from build123d import *

# Parameters (mm, degrees)
CROQUIS1_W              = 5
CROQUIS1_H              = 35
SALIENTE_EXTRUIR2_DEPTH = 5


with BuildPart() as part:
    # Croquis1 → Saliente-Extruir2 (new body)
    with BuildSketch(Plane(origin=(0, 0, 0), x_dir=(1, 0, 0), z_dir=(0, 1, 0))):
        with BuildLine():
            Line((-40, -25), (40, -25))
            ThreePointArc((40, -25), (47.071067812, -22.071067812), (50, -15))
            Line((50, -15), (50, 15))
            ThreePointArc((50, 15), (47.071067812, 22.071067812), (40, 25))
            Line((40, 25), (-40, 25))
            ThreePointArc((-40, 25), (-47.071067812, 22.071067812), (-50, 15))
            Line((-50, 15), (-50, -15))
            ThreePointArc((-50, -15), (-47.071067812, -22.071067812), (-40, -25))
        make_face()
        with Locations((-45, 0)):
            Rectangle(CROQUIS1_W, CROQUIS1_H, mode=Mode.SUBTRACT)
        with Locations((45, 0)):
            Rectangle(CROQUIS1_W, CROQUIS1_H, mode=Mode.SUBTRACT)
    extrude(amount=SALIENTE_EXTRUIR2_DEPTH)


solid = part.part
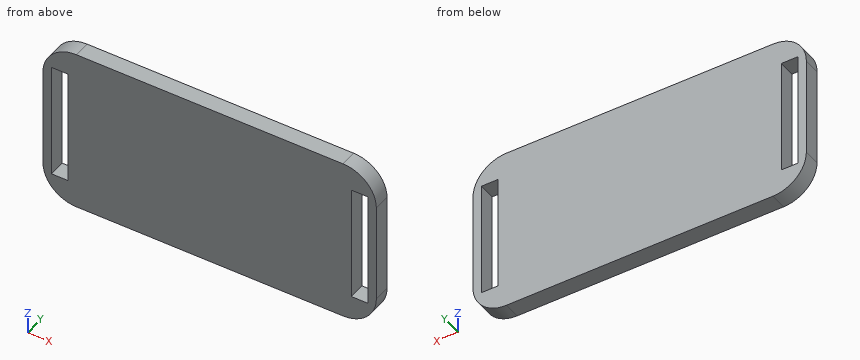
Input: part model. Units: mm. Frame: model coordinates. Coordinates: 2 decimals unless noted, no trailing zeros. Order: outer loops, then holes, each group sorted by start corner. A loop starts at its lowest first (then second) coordinate and runs counter-clockwise, first axis right, second up. Notation, with made-up numbers: M 13.25,46 L 57.25,46 A9 cw 57.25,61 Z; hole C -5,70.25 d10. An arc over 180 degrees is marked long. Answer in a Markdown table with one row per item.
(1) Material intervals for line 1 (X direction, y = 2.6, z = 2); line 2 (X direction, y = 1.9, z = 17); line 3 (Z direction, x = 43.5, y = 4.85), sorted ascending. Write a range as [from, to].
Numbers:
| item | result |
|---|---|
| line 1 | x = [-50, -47.5], [-42.5, 42.5], [47.5, 50] |
| line 2 | x = [-49.8, -47.5], [-42.5, 42.5], [47.5, 49.8] |
| line 3 | z = [-24.37, -17.5], [17.5, 24.37] |
(2) Section query C-C, the plane z = -16.5. Output: boundary loops of the cut face in (x, y), plus the area to 3 significant figures.
Numbers:
| item | result |
|---|---|
| outline | M -49.89,0 L -47.5,0 L -47.5,5 L -49.89,5 Z; M -42.5,0 L 42.5,0 L 42.5,5 L -42.5,5 Z; M 47.5,0 L 49.89,0 L 49.89,5 L 47.5,5 Z |
| area | 449 mm^2 |
(3) Section query B-B, the plane y = 2.2. Output: boundary loops of the cut face in (x, z), plus the area to 3 significant figures.
Numbers:
| item | result |
|---|---|
| outline | M -50,-15 A10 ccw -40,-25 L 40,-25 A10 ccw 50,-15 L 50,15 A10 ccw 40,25 L -40,25 A10 ccw -50,15 Z; hole M -47.5,-17.5 L -42.5,-17.5 L -42.5,17.5 L -47.5,17.5 Z; hole M 42.5,-17.5 L 47.5,-17.5 L 47.5,17.5 L 42.5,17.5 Z |
| area | 4,560 mm^2 |
(4) Section query A-A, the plane z = 10. Output: boundary loops of the cut face in (x, y), plus the area to 3 significant figures.
Numbers:
| item | result |
|---|---|
| outline | M -50,0 L -47.5,0 L -47.5,5 L -50,5 Z; M -42.5,0 L 42.5,0 L 42.5,5 L -42.5,5 Z; M 47.5,0 L 50,0 L 50,5 L 47.5,5 Z |
| area | 450 mm^2 |
(5) Contact query for flat-ended pins moving along their axis: pin 1 Ø2.5 at (x, y) = (45, 3) entering from +Z; pin 2 Ø1.5 at (x, y) = (-45, 1.5) entering from -Z; pin 3 Ø1.5 at (y, z) = (2, -19) entering from +X. Output: stop coordinate, or through.
Numbers:
| item | result |
|---|---|
| pin 1 | stops at z = 24.27 |
| pin 2 | stops at z = -24.05 |
| pin 3 | stops at x = 49.46 |
(6) Section query D-D, the plane z = 20. Output: boundary loops of the cut face in (x, y).
Numbers:
| item | result |
|---|---|
| outline | M -48.66,0 L 48.66,0 L 48.66,5 L -48.66,5 Z |
